Model file for the job. Use its own axes, mm. A direction names the side the tool comes from. Round coordinates to 2 decimals unless told otherwise and drop trailing zeros. Order: outer loops, then holes, each group sorted by start corner. A loop starts at its lowest first (then second) coordinate and runs counter-clockwise, first axis right, second up. Notation, with made-up numbers: M 73.25,70.25 L 123.25,70.25 A17 ccw 123.25,86.25 Z; hole C 33.25,22.25 d5. An arc over 180 degrees is marked long. Return JSON: item names as keys, results as strings. Group by question number.
Item 1: Slice it at A-A on y = -1.05. Write the cut outline in (x, z).
Item 2: Pull direction Z, two halves, no side cores. Call faces 4 (the face through (-63, -1, 15)), 5 (the face through (-67.78, -1.23, 21.64)), 6 (the face through (-35, -2.5, 3)), 7 (the face through (-54, -3, -11)): pulls with the +Z half, pulls with the -Z half, needs draft (parallel to the pull), parting line crosses it, or undercut.
Item 3: Slice it at C-C on z = -26. Write the cut outline in (x, y), then the cut area to 3 significant figures.
Item 4: Slice it at B-B on z = 7. Write the cut outline in (x, y).
Item 5: Pin check, flat tips, straight feed: pin 1 Ø2.5 at (x, y) = (-27.94, -4) entering from -Z; pin 2 Ø2 at (x, y) = (-32.5, -1) entering from +Z; pin 3 Ø1.5 at (y, z) = (-4, -30) entering from -X. Stop position of each tip, or through.
Item 6: Which spindle directions (+Z, -Z, +X, -X, +Y, -Y) get a long thin tool onto all of the face, cutting with end or side? Do faces 1 (the face through (-51.77, -3.98, -39.34)), 2 (the face through (-54, -4, 10)), 3 (the face through (-64.6, -1.23, 22.25)). Say none if no direction does.
Item 7: Probe line 1 along Z through (x, y) = (-4, -4.7) (3 decimals); line 2 along Z through (x, y) = (-50, -4.9) (3 decimals); line 3 along Z through (x, y) = (-8, -3.5). List the from-to ranges inside material, lowest first.
from build123d import *

# Parameters (mm, degrees)
F1_DEPTH  = 5.5
F3_DEPTH  = 3
F4_R      = 0.5
F5_DEPTH  = 1.125
F9_DEPTH  = 12.5
F10_W     = 14.8
F10_H     = 2.5
F11_DEPTH = 47
F13_DEPTH = 13.5
F14_R     = 0.5
F15_DEPTH = 4.25
F16_R     = 1
F17_DEPTH = 4.25


with BuildPart() as f1:
    # F0 (on Front) → F1 (new body)
    with BuildSketch(Plane.XZ):
        with BuildLine():
            Line((0, -12.5), (0, 12.5))
            Line((0, 12.5), (-63, 12.5))
            Line((-63, 12.5), (-63, 19))
            ThreePointArc((-63, 19), (-62.7071067812, 19.7071067812), (-62, 20))
            Line((-62, 20), (-62, 29.5))
            ThreePointArc((-62, 29.5), (-67.1049806801, 23.2039800052), (-68.93, 15.3065120566))
            Line((-68.93, 15.3065120566), (-68.93, -2.5))
            Line((-68.93, -2.5), (-54, -2.5))
            Line((-54, -2.5), (-54, -19.0381197846))
            Line((-54, -19.0381197846), (-54.8, -19.5))
            Line((-54.8, -19.5), (-54.8, -47.5))
            Line((-54.8, -47.5), (-48.1705947427, -44.1845815863))
            Line((-48.1705947427, -44.1845815863), (-40, -12.5))
            Line((-40, -12.5), (0, -12.5))
        make_face()
    extrude(amount=F1_DEPTH)

    # F2 (on face) → F3 (cut)
    with BuildSketch(Plane.XZ.offset(5.5)):
        Polygon((0, -8.25), (0, 8.25), (-54, 8.25), (-54, 31.9336503744), (-73.7788975239, 31.9336503744), (-73.7788975239, -2.5), (-54, -2.5), (-54, -8.25), align=None)
    extrude(amount=-F3_DEPTH, mode=Mode.SUBTRACT)

    # F4 (on face) → F5 (cut)
    with BuildSketch(Plane.XZ.offset(5.5)):
        with Locations((-4, 10.375)):
            Circle(F4_R)
        with Locations((-27, 10.375)):
            Circle(F4_R)
        with Locations((-50, 10.375)):
            Circle(F4_R)
        with Locations((-50, -10.375)):
            Circle(F4_R)
        with Locations((-27, -10.375)):
            Circle(F4_R)
        with Locations((-4, -10.375)):
            Circle(F4_R)
    extrude(amount=-F5_DEPTH, mode=Mode.SUBTRACT)

    # F8 (on offset) → F9 (cut)
    with BuildSketch(Plane.XY.offset(30)):
        Polygon((-67.1257596039, 0), (-62, -2.5), (-62, 0), align=None)
    extrude(amount=-F9_DEPTH, mode=Mode.SUBTRACT)

    # F10 (on face) → F11 (cut)
    with BuildSketch(Plane(origin=(0, 0, -12.5), x_dir=(1, 0, 0), z_dir=(0, 0, -1))):
        with Locations((-47.4, 1.25)):
            Rectangle(F10_W, F10_H)
    extrude(amount=F11_DEPTH, mode=Mode.SUBTRACT)

    # F12 (on plane+point) → F13 (cut)
    with BuildSketch(Plane(origin=(0, 0, -47.5), x_dir=(1, 0, 0), z_dir=(0, 0, -1))):
        Polygon((-48.6490884753, 5.5), (-54.8, 5.5), (-54.8, 2.5), align=None)
    extrude(amount=-F13_DEPTH, mode=Mode.SUBTRACT)

    # F14 (on face) → F15 (cut, through all)
    with BuildSketch(Plane.XY.offset(12.5)):
        with Locations((-7.54, -4)):
            Circle(F14_R)
        with Locations((-48.34, -4)):
            Circle(F14_R)
    extrude(amount=-F15_DEPTH, mode=Mode.SUBTRACT)

    # F16 (on face) → F17 (cut, through all)
    with BuildSketch(Plane.XY.offset(12.5)):
        with Locations((-27.94, -4)):
            Circle(F16_R)
    extrude(amount=-F17_DEPTH, mode=Mode.SUBTRACT)


solid = f1.part
Output values:
{
 "1": {"outline": "M -68.93,-2.5 L -54,-2.5 L -54,-12.5 L 0,-12.5 L 0,12.5 L -63,12.5 L -63,17.5 L -64.97,17.5 L -64.97,26.57 A18 ccw -68.93,15.31 Z"},
 "2": {"face 4": "undercut", "face 5": "pulls with the +Z half", "face 6": "undercut", "face 7": "needs draft"},
 "3": {"outline": "M -54.8,-5.5 L -43.48,-5.5 L -43.48,-2.5 L -54.8,-2.5 Z", "area": "34.0 mm²"},
 "4": {"outline": "M -68.93,-2.5 L 0,-2.5 L 0,0 L -68.93,0 Z"},
 "5": {"pin 1": "z = -12.5", "pin 2": "z = 12.5", "pin 3": "x = -54.8"},
 "6": {"face 1": "-Z, -X, -Y", "face 2": "+Z, -X, -Y", "face 3": "+Z, +X, +Y"},
 "7": {"line 1": "-12.5 to -10.875, -9.875 to -8.25, 8.25 to 9.875, 10.875 to 12.5", "line 2": "-34 to -10.875, -9.875 to -8.25, 8.25 to 9.875, 10.875 to 12.5", "line 3": "-12.5 to -8.25, 8.25 to 12.5"}
}
